Here's how the part is built. I have some questions about the finished solid (model axes, mm). A direction names the side the tool comes from. Coordinates: 2 decimals unless noted, no trailing zeros. Write each loop counter-clockwise with the first axis right and the second up, starting at its lowest first coordinate (ties: lowest second). Pieces come first, ordered by that corner, then holes.
Item 1: Please list where these lines run through material, in increasing order: line 1 (Y direction, x = -47.5, z = -47.5); line 2 (Z direction, x = -44.5, y = 348); line 3 (X direction, y = 328, z = 9).
Item 2: I want a section at B-B (y = 45). Please give me the cut outline in (x, z), and give its area (3 significant figures).
Item 3: If we mould it in two halves opening along Z, with no side actions, what happens to faces 3 (the face through (-53, 419, -93)), 4 (the face through (-42.154, 804.56, 102.495)), 5 (the face through (-9, 419, 112.5))? For each: pulls with the +Z half, pulls with the -Z half, needs draft (parallel to the pull), parting line crosses it, or undercut.
Item 4: For faces 1 (the face through (-42, 25, 33)), 2 (the face through (-53, 837, 32)), which set-ups out of +Z, -Z, +X, -X, +Y, -Y let a thin tool reach every point of the face, with its end or its side?
from build123d import *

# Parameters (mm, degrees)
BOSS_EXTRUDE1_DEPTH = 850
CUT_EXTRUDE1_DEPTH  = 22


with BuildPart() as part:
    # Sketch1 → Boss-Extrude1 (new body)
    with BuildSketch(Plane(origin=(0, 0, 0), x_dir=(1, 0, 0), z_dir=(0, 1, 0))):
        Polygon((-53, -73), (-53, -112.5), (37, -112.5), (37, -84), (53, -100), (53, 100), (37, 84), (37, 112.5), (-53, 112.5), (-53, 73), (-43, 73), (-43, 77.5), (-31, 77.5), (-31, 52.5), (-43, 52.5), (-43, 57), (-53, 57), (-53, 8), (-43, 8), (-43, 12.5), (-31, 12.5), (-31, -12.5), (-43, -12.5), (-43, -8), (-53, -8), (-53, -57), (-43, -57), (-43, -52.5), (-31, -52.5), (-31, -77.5), (-43, -77.5), (-43, -73), align=None)
    extrude(amount=BOSS_EXTRUDE1_DEPTH)

    # Sketch2 → Cut-Extrude1 (cut)
    with BuildSketch(Plane.ZY.offset(53)):
        with BuildLine():
            Line((-82.5, 65), (82.5, 65))
            ThreePointArc((82.5, 65), (102.5, 45), (82.5, 25))
            Line((82.5, 25), (-82.5, 25))
            ThreePointArc((-82.5, 25), (-102.5, 45), (-82.5, 65))
        make_face()
        with BuildLine():
            Line((-82.5, 785), (82.5, 785))
            ThreePointArc((82.5, 785), (102.5, 805), (82.5, 825))
            Line((82.5, 825), (-82.5, 825))
            ThreePointArc((-82.5, 825), (-102.5, 805), (-82.5, 785))
        make_face()
    extrude(amount=-CUT_EXTRUDE1_DEPTH, mode=Mode.SUBTRACT)


solid = part.part
Answer:
1. line 1: y = 0 to 25, 65 to 785, 825 to 850
1. line 2: z = -112.5 to -73, -57 to -8, 8 to 57, 73 to 112.5
1. line 3: x = -53 to -43, -31 to 53
2. outline: (-53, -112.5) - (37, -112.5) - (37, -84) - (53, -100) - (53, 100) - (37, 84) - (37, 112.5) - (-53, 112.5) - (-53, 102.5) - (-31, 102.5) - (-31, -102.5) - (-53, -102.5) - close
2. area: 18,700 mm2
3. face 3: needs draft
3. face 4: undercut
3. face 5: pulls with the +Z half
4. face 1: -X
4. face 2: +Z, -Z, -X, +Y, -Y
